Can you work these out from the drawing? Everything is in mm from the part's minimum corner. A direction names the side the tool comes from. Coordinates: 2 decimals unless noted, no trailing zeros. Loops run counter-clockwise (first coordinate to the right, second up) from the corner with the lowest first, then second, coordinate; pieces in that order, holes last.
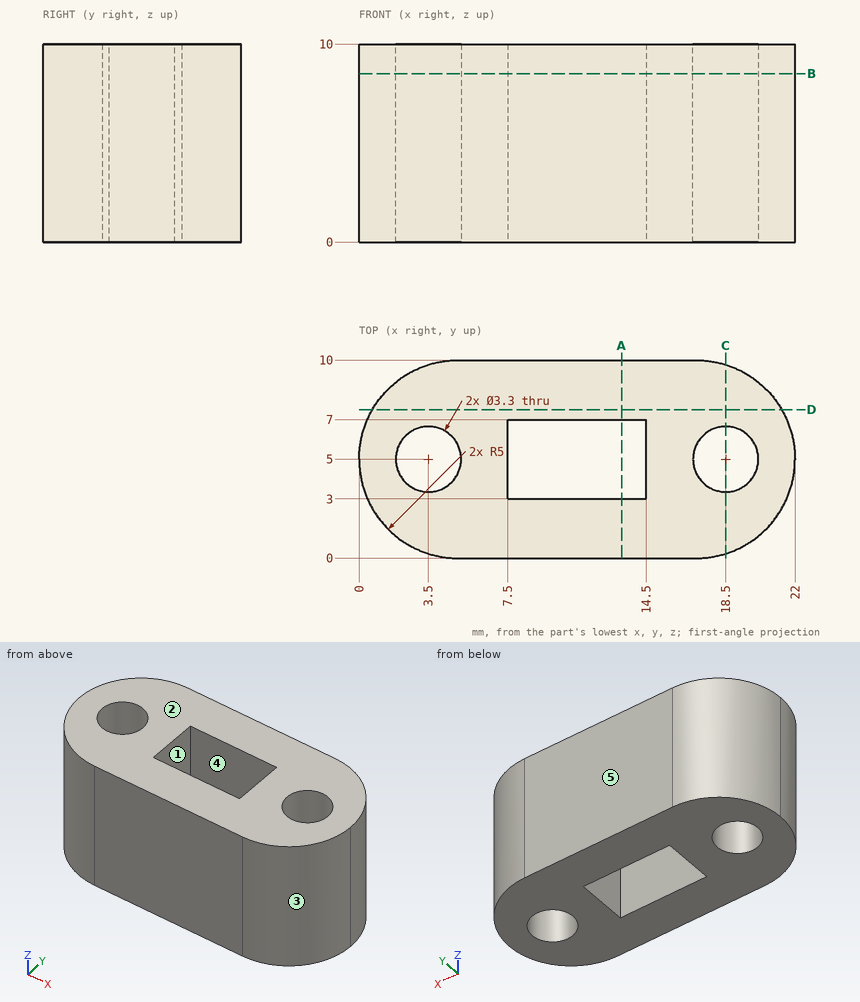
(1) Imagine slicing it at D-D, the plane y = 7.5. Write out the boundary of the cut face in (x, z).
Answers:
outline: (0.67, 0) - (21.33, 0) - (21.33, 10) - (0.67, 10) - close
(2) Imagine slicing it at A-A, the plane x = 13.25. Write out the boundary of the cut face in (y, z).
Answers:
outline: (0, 0) - (3, 0) - (3, 10) - (0, 10) - close; (7, 0) - (10, 0) - (10, 10) - (7, 10) - close
(3) Imagine slicing it at C-C, the plane x = 18.5. Write out the boundary of the cut face in (y, z).
Answers:
outline: (0.23, 0) - (3.35, 0) - (3.35, 10) - (0.23, 10) - close; (6.65, 0) - (9.77, 0) - (9.77, 10) - (6.65, 10) - close
(4) For pin 1 (2 mm diameter, centred on x = 3, z = 2, fed in from -Y); pin 2 (3 mm diameter, centred on x = 3.5, y = 5, fed in from -Z); pin 3 (1 mm diameter, centred on y = 6, z = 6, fed in from -X), each with a flat end and sliding along its axis, tell me the tip position at first contact or that it passes through.
Answers:
pin 1: stops at y = 0.1
pin 2: passes through
pin 3: stops at x = 0.03
(5) Imagine slicing it at B-B, the plane z = 8.5. State how many separate pieces and enclosed holes the cut face has, and give its area (3 significant figures).
Answers:
separate pieces: 1
enclosed holes: 3
area: 153 mm2
(6) We'd pull the mould along X, two halves only. Please class the marked faces 3, 4 and 5: +X half, -X half, draft (parallel to the pull), parting line (faces both ways), or undercut.
Answers:
face 3: +X half
face 4: undercut
face 5: draft
(7) Which directions (+Z, -Z, +X, -X, +Y, -Y) give clear straight access to the entire face, cutting with the end or side of a thin tool? Please do the marked faces 1 and 2.
Answers:
face 1: +Z, -Z
face 2: +Z, +X, -X, +Y, -Y
(8) I need wall thicknesses on probe 1 along Y at (x, z) = (11, 1.5); probe 2 along X at (y, z) = (4.25, 3.5); probe 3 along X at (y, z) = (4.75, 4). Which ranges of each line are inside material? Lowest first, please.
Answers:
probe 1: y = 0 to 3, 7 to 10
probe 2: x = 0.06 to 2.03, 4.97 to 7.5, 14.5 to 17.03, 19.97 to 21.94
probe 3: x = 0.01 to 1.87, 5.13 to 7.5, 14.5 to 16.87, 20.13 to 21.99
